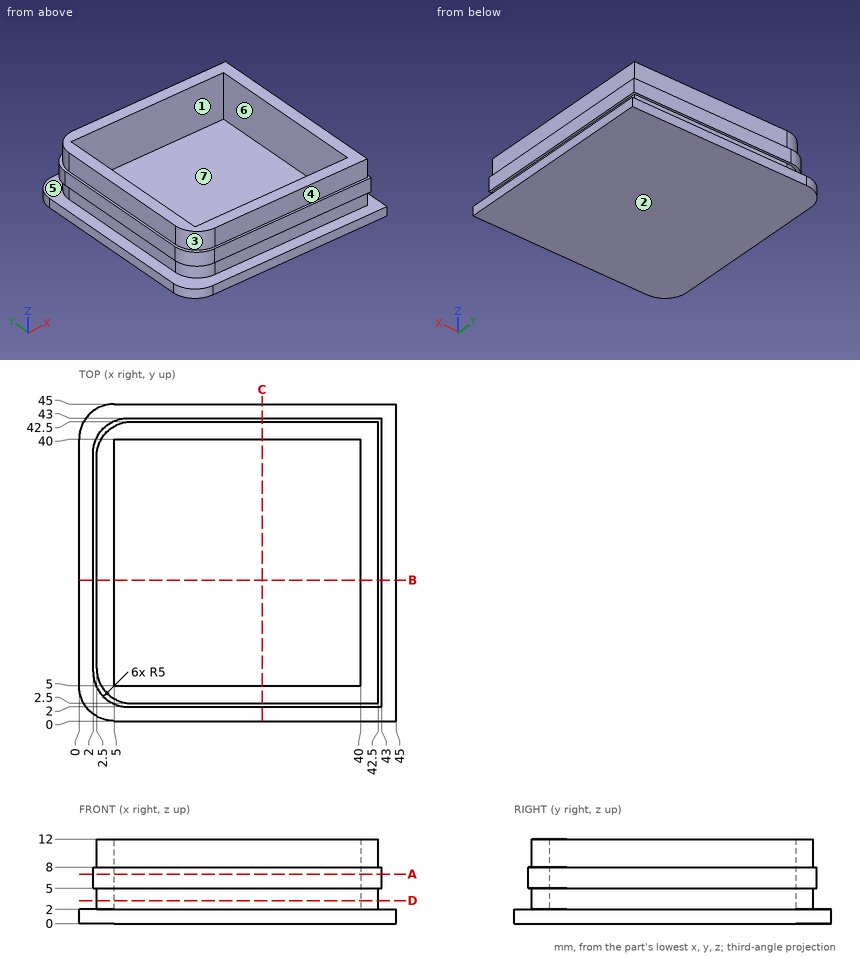
Design review of the part shown in the three views and the two pictorial views. Dimensions are in mm from the part's minimum x, y and z. A direction names the side the tool comes from. Give positions to 0.01 mm unless a question says otherwise; leave off trailing zeros. Write each loop counter-clockwise with the first axis right and the second up, starting at its lowest first coordinate (ties: lowest second). Pieces come first, ordered by that corner, then holes. Notation, with made-up numbers: (82.25, 6) - (103.25, 6) arc R8 ccw to (103.25, 19) - close; hole circle Ø8 at (65, 61.25). An arc over 180 degrees is marked (long way). Return JSON: item names as keys, results as strings. Group by question number.
(1) We need section A-A, the plane z = 7. Give the boundary of the cut face in (x, y), then the cut area to 3 significant figures.
(2) We need section D-D, the plane z = 3.25. Give the boundary of the cut face in (x, y).
(3) Machinability: for the marked faces 1, 2, 3 and 4, which of the approach directions +Z, -Z, +X, -X, +Y, -Y give a long, thin tool a straight path to every point of the face, cutting with its end or side? Answer none if there is none.
(4) To check wall thickness, follow probe 1 along X at (y, z) = (9, 6.25); probe 2 along X at (y, z) = (35, 11.75). State the ranges of each line that lie inside material, in increasing order.
(5) Insertion check: pin 1 (22.5 mm diameter, centred on x = 19.5, y = 26, fed in from +Z); pin 2 (1.2 mm diameter, centred on x = 26, z = 10, fed in from +Y); pin 3 (4.5 mm diameter, centred on x = 26, z = 10, fed in from -Y). Each pin has a flat end and moves straight along its axis. Give the tip position at first contact, or say it passes through.
(6) Mouldability with a two-part tool opening along Z and no side actions: class the marked faces 5, 6 and 7 as +Z half, -Z half, draft (parallel to the pull), parting line (faces both ways), or undercut.
(7) We need section B-B, the plane y = 20. Give the boundary of the cut face in (x, z).
Reported:
{
 "1": {"outline": "(2, 7) arc R5 ccw to (7, 2) - (43, 2) - (43, 43) - (7, 43) arc R5 ccw to (2, 38) - close; hole (5, 5) - (40, 5) - (40, 40) - (5, 40) - close", "area": "445 mm2"},
 "2": {"outline": "(2.5, 7.5) arc R5 ccw to (7.5, 2.5) - (42.5, 2.5) - (42.5, 42.5) - (7.5, 42.5) arc R5 ccw to (2.5, 37.5) - close; hole (5, 5) - (40, 5) - (40, 40) - (5, 40) - close"},
 "3": {"face 1": "+Z", "face 2": "-Z, +X, -X, +Y, -Y", "face 3": "+Z, -X, -Y", "face 4": "+Z, +X, -X, -Y"},
 "4": {"probe 1": "x = 2 to 5, 40 to 43", "probe 2": "x = 2.5 to 5, 40 to 42.5"},
 "5": {"pin 1": "stops at z = 2", "pin 2": "stops at y = 42.5", "pin 3": "stops at y = 2"},
 "6": {"face 5": "undercut", "face 6": "draft", "face 7": "+Z half"},
 "7": {"outline": "(0, 0) - (45, 0) - (45, 2) - (42.5, 2) - (42.5, 5) - (43, 5) - (43, 8) - (42.5, 8) - (42.5, 12) - (40, 12) - (40, 2) - (5, 2) - (5, 12) - (2.5, 12) - (2.5, 8) - (2, 8) - (2, 5) - (2.5, 5) - (2.5, 2) - (0, 2) - close"}
}
